Geometry: final body of the model. Coordinates: model frame, mm. Give positions to 0.01 mm unless a question says otherwise; leave off trailing zeros. Loops run counter-clockwise (first coordinate to the right, second up) from the corner with the lowest first, then second, coordinate; pieces in that order, holes last.
from build123d import *

# Parameters (mm, degrees)
F1_DEPTH = 0.762


with BuildPart() as f1:
    # F0 (on Top) → F1 (new body)
    with BuildSketch(Plane.XY):
        with BuildLine():
            ThreePointArc((0, 24.384), (0.853544, -24.369057), (-1.706041, 24.324245))
            Line((-1.706041, 24.324245), (-1.768951, 25.221201))
            ThreePointArc((-1.768951, 25.221201), (-0.10991, -25.282921), (1.988164, 25.204868))
            Line((1.988164, 25.204868), (2.05887, 26.101239))
            Line((2.05887, 26.101239), (-3.534211, 26.542422))
            Line((-3.534211, 26.542422), (-3.609026, 25.646375))
            Line((-3.609026, 25.646375), (0, 25.361695))
            Line((0, 25.361695), (0, 24.384))
        make_face()
    extrude(amount=F1_DEPTH)


solid = f1.part
Item 1: Ray query, probe 1 along X at (y, z) = (0, 0.35); probe 2 along Y at (x, z) = (21, 0.4); probe 3 along Y at (x, z) = (-6, 0.5). Return the intervals inside material, ascending.
Values follow:
probe 1: x = -25.28 to -24.38, 24.38 to 25.28
probe 2: y = -14.08 to -12.39, 12.39 to 14.08
probe 3: y = -24.56 to -23.63, 23.63 to 24.56
Item 2: Section query C-C on z = 0.25. Return loops of the section in (x, y).
Values follow:
outline: (-3.61, 25.65) - (0, 25.36) - (0, 24.38) arc R24.38 cw (long way) to (-1.71, 24.32) - (-1.77, 25.22) arc R25.28 ccw (long way) to (1.99, 25.2) - (2.06, 26.1) - (-3.53, 26.54) - close
Item 3: Draft query along Y for faces 1 (the face through (6, 24, 0.762)), 2 (the face through (1.91, -24.31, 0.38)). Return one class per face: +Y half, -Y half, draft (parallel to the pull), parting line (faces both ways), or undercut.
Values follow:
face 1: draft
face 2: undercut
Item 4: Section query A-A on y = 0. Return loops of the section in (x, z).
Values follow:
outline: (-25.28, 0) - (-24.38, 0) - (-24.38, 0.76) - (-25.28, 0.76) - close; (24.38, 0) - (25.28, 0) - (25.28, 0.76) - (24.38, 0.76) - close
Item 5: Section query B-B on x = 5.5. Return loops of the section in (y, z).
Values follow:
outline: (-24.68, 0) - (-23.76, 0) - (-23.76, 0.76) - (-24.68, 0.76) - close; (23.76, 0) - (24.68, 0) - (24.68, 0.76) - (23.76, 0.76) - close
